Geometry check sheet. Reference: the model listing, model coordinates, mm. A direction names the side the tool comes from. Round coordinates to 2 decimals unless told otherwise and drop trailing zeros. Write each loop counter-clockwise with the first axis right and the second up, starting at its lowest first coordinate (ties: lowest second). Pieces come first, ordered by that corner, then holes. Notation, with made-up numbers: (12.25, 82) - (20.25, 82) arc R33 ccw to (20.25, 115) - close; hole circle Ø5 at (2, 18). An arc over 180 degrees is marked (long way). Return JSON: item names as keys, results as strings.
```python
from build123d import *

# Parameters (mm, degrees)
F0_W     = 127.8
F0_H     = 85.4
F1_DEPTH = 5
F2_R     = 2.4425
F3_DEPTH = 25


with BuildPart() as f1:
    # F0 (on Top) → F1 (new body)
    with BuildSketch(Plane.XY):
        Rectangle(F0_W, F0_H)
    extrude(amount=F1_DEPTH)

    # F2 (on face) → F3 (join)
    with BuildSketch(Plane.XY.offset(5)):
        with Locations((-57.592481, 35.563733)):
            Circle(F2_R)
        with Locations((-44.592481, 35.563733)):
            Circle(F2_R)
        with Locations((-31.592481, 35.563733)):
            Circle(F2_R)
        with Locations((-18.592481, 35.563733)):
            Circle(F2_R)
        with Locations((-5.592481, 35.563733)):
            Circle(F2_R)
        with Locations((7.407519, 35.563733)):
            Circle(F2_R)
        with Locations((20.407519, 35.563733)):
            Circle(F2_R)
        with Locations((33.407519, 35.563733)):
            Circle(F2_R)
        with Locations((46.407519, 35.563733)):
            Circle(F2_R)
        with Locations((59.407519, 35.563733)):
            Circle(F2_R)
        with Locations((46.407519, 22.563733)):
            Circle(F2_R)
        with Locations((33.407519, 22.563733)):
            Circle(F2_R)
        with Locations((59.407519, 22.563733)):
            Circle(F2_R)
        with Locations((-57.592481, 22.563733)):
            Circle(F2_R)
        with Locations((-44.592481, 22.563733)):
            Circle(F2_R)
        with Locations((-31.592481, 22.563733)):
            Circle(F2_R)
        with Locations((-18.592481, 22.563733)):
            Circle(F2_R)
        with Locations((-5.592481, 22.563733)):
            Circle(F2_R)
        with Locations((7.407519, 22.563733)):
            Circle(F2_R)
        with Locations((20.407519, 22.563733)):
            Circle(F2_R)
        with Locations((46.407519, 9.563733)):
            Circle(F2_R)
        with Locations((33.407519, 9.563733)):
            Circle(F2_R)
        with Locations((59.407519, 9.563733)):
            Circle(F2_R)
        with Locations((-57.592481, 9.563733)):
            Circle(F2_R)
        with Locations((-44.592481, 9.563733)):
            Circle(F2_R)
        with Locations((-31.592481, 9.563733)):
            Circle(F2_R)
        with Locations((-18.592481, 9.563733)):
            Circle(F2_R)
        with Locations((-5.592481, 9.563733)):
            Circle(F2_R)
        with Locations((7.407519, 9.563733)):
            Circle(F2_R)
        with Locations((20.407519, 9.563733)):
            Circle(F2_R)
        with Locations((46.407519, -3.436267)):
            Circle(F2_R)
        with Locations((33.407519, -3.436267)):
            Circle(F2_R)
        with Locations((59.407519, -3.436267)):
            Circle(F2_R)
        with Locations((-57.592481, -3.436267)):
            Circle(F2_R)
        with Locations((-44.592481, -3.436267)):
            Circle(F2_R)
        with Locations((-31.592481, -3.436267)):
            Circle(F2_R)
        with Locations((-18.592481, -3.436267)):
            Circle(F2_R)
        with Locations((-5.592481, -3.436267)):
            Circle(F2_R)
        with Locations((7.407519, -3.436267)):
            Circle(F2_R)
        with Locations((20.407519, -3.436267)):
            Circle(F2_R)
        with Locations((46.407519, -16.436267)):
            Circle(F2_R)
        with Locations((33.407519, -16.436267)):
            Circle(F2_R)
        with Locations((59.407519, -16.436267)):
            Circle(F2_R)
        with Locations((-57.592481, -16.436267)):
            Circle(F2_R)
        with Locations((-44.592481, -16.436267)):
            Circle(F2_R)
        with Locations((-31.592481, -16.436267)):
            Circle(F2_R)
        with Locations((-18.592481, -16.436267)):
            Circle(F2_R)
        with Locations((-5.592481, -16.436267)):
            Circle(F2_R)
        with Locations((7.407519, -16.436267)):
            Circle(F2_R)
        with Locations((20.407519, -16.436267)):
            Circle(F2_R)
        with Locations((46.407519, -29.436267)):
            Circle(F2_R)
        with Locations((33.407519, -29.436267)):
            Circle(F2_R)
        with Locations((59.407519, -29.436267)):
            Circle(F2_R)
        with Locations((-57.592481, -29.436267)):
            Circle(F2_R)
        with Locations((-44.592481, -29.436267)):
            Circle(F2_R)
        with Locations((-31.592481, -29.436267)):
            Circle(F2_R)
        with Locations((-18.592481, -29.436267)):
            Circle(F2_R)
        with Locations((-5.592481, -29.436267)):
            Circle(F2_R)
        with Locations((7.407519, -29.436267)):
            Circle(F2_R)
        with Locations((20.407519, -29.436267)):
            Circle(F2_R)
    extrude(amount=F3_DEPTH)


solid = f1.part
```
(1) Section check A-A, the plane x = -32.5. Enter the section's corners in (y, z), plus the area to 3 significant figures.
Response values:
{"outline": "(-42.7, 0) - (42.7, 0) - (42.7, 5) - (37.83, 5) - (37.83, 30) - (33.3, 30) - (33.3, 5) - (24.83, 5) - (24.83, 30) - (20.3, 30) - (20.3, 5) - (11.83, 5) - (11.83, 30) - (7.3, 30) - (7.3, 5) - (-1.17, 5) - (-1.17, 30) - (-5.7, 30) - (-5.7, 5) - (-14.17, 5) - (-14.17, 30) - (-18.7, 30) - (-18.7, 5) - (-27.17, 5) - (-27.17, 30) - (-31.7, 30) - (-31.7, 5) - (-42.7, 5) - close", "area": "1,110 mm^2"}
(2) Access from +Z, -Z, +X, -X, +Y, -Y to the whole of each face (thin tool, end or side, straight path). Record for faces 1 (the face through (45.88, 33.18, 17.32)), 2 (the face through (20, -3, 30)).
Response values:
{"face 1": "+Z", "face 2": "+Z, +X, -X, +Y, -Y"}
(3) Section check C-C, the plane z = 22.5. Give the number of separate pieces and of enclosed holes in the cut face, plus the area to 3 significant figures.
Response values:
{"separate pieces": "60", "enclosed holes": "0", "area": "1,120 mm^2"}
(4) Material ranges on line 1 along Z through (x, y) = (3, 6); line 2 along Y through (x, z) = (-6.5, 25.5); line 3 along Y through (x, z) = (-18, 21.25), recorded low to high. Write a range as [from, to].
Response values:
{"line 1": "z = [0, 5]", "line 2": "y = [-31.7, -27.17], [-18.7, -14.17], [-5.7, -1.17], [7.3, 11.83], [20.3, 24.83], [33.3, 37.83]", "line 3": "y = [-31.81, -27.07], [-18.81, -14.07], [-5.81, -1.07], [7.19, 11.93], [20.19, 24.93], [33.19, 37.93]"}
(5) Gauge pin test, flat ends, axial feed: pin 1 (3 mm diameter, centred on x = 31, y = 9, fed in from -Z); pin 2 (2 mm diameter, centred on y = -32.5, z = 12.5, fed in from +X); pin 3 (10 mm diameter, centred on x = -33.5, z = 20, fed in from -Y); pin 4 (10 mm diameter, centred on y = 21, z = 16.5, fed in from +X). Record the tip position at first contact, or that the pin passes through.
Response values:
{"pin 1": "stops at z = 0", "pin 2": "stops at x = 60.71", "pin 3": "stops at y = -31.88", "pin 4": "stops at x = 61.85"}
(6) Release check for a two-part mould opening along X. For faces 3 (the face through (6.88, -5.82, 17.32)), 4 (the face through (20, 36, 30)) record: pulls with the +X half, pulls with the -X half, needs draft (parallel to the pull), parting line crosses it, or undercut.
Response values:
{"face 3": "undercut", "face 4": "needs draft"}
(7) Section check B-B, the plane y = 14.5. Enter the section's corners in (x, z), plus the area to 3 significant figures.
Response values:
{"outline": "(-63.9, 0) - (63.9, 0) - (63.9, 5) - (-63.9, 5) - close", "area": "639 mm^2"}
